```python
from build123d import *

# Parameters (mm, degrees)
SKETCH1_W                        = 12.7
SKETCH1_H                        = 6.0198
BOSS_EXTRUDE1_DEPTH              = 5.7658
SKETCH13_R                       = 0.635
CUT_EXTRUDE2_DEPTH               = 5.7658
CHAMFER1_SIZE                    = 50.8
F_4_CLEARANCE_HOLE1_D            = 2.9464
F_4_CLEARANCE_HOLE1_DEPTH        = 6.35
F_4_CLEARANCE_HOLE1_TIP          = 0.885187864
F_3_8_0_375_DIAMETER_HOLE1_D     = 9.525
F_3_8_0_375_DIAMETER_HOLE1_DEPTH = 6.35
F_3_8_0_375_DIAMETER_HOLE1_TIP   = 2.861598698
CUT_EXTRUDE3_REACH               = 234.708
FILLET3_R                        = 6.35
CUT_EXTRUDE4_REACH               = 234.708
CUT_EXTRUDE5_REACH               = 234.708
SKETCH26_W                       = 2.9591
SKETCH26_H                       = 9.525
CUT_EXTRUDE6_REACH               = 234.708
SKETCH29_W                       = 65.024
SKETCH29_H                       = 36.83
FILLET5_R                        = 6.35
CUT_EXTRUDE9_REACH               = 234.708
SKETCH32_W                       = 9.525
SKETCH32_H                       = 2.9591
CUT_EXTRUDE10_REACH              = 234.708
CHAMFER2_SIZE                    = 19.05
CUT_EXTRUDE11_START              = -5.7658
CUT_EXTRUDE11_DEPTH              = 5.7658
CUT_EXTRUDE12_REACH              = 234.708
SKETCH36_W                       = 57.277
SKETCH36_H                       = 36.83
FILLET7_R                        = 2.54
FILLET8_R                        = 6.35
CUT_EXTRUDE13_REACH              = 234.708
SKETCH37_W                       = 9.525
SKETCH37_H                       = 2.9591
F_4_CLEARANCE_HOLE2_D            = 2.9464
F_4_CLEARANCE_HOLE2_DEPTH        = 5.7658
SKETCH38_W                       = 50.8
SKETCH38_H                       = 19.05
CUT_EXTRUDE14_DEPTH              = 233.70795425
FILLET9_R                        = 6.35
TAP_DRILL_FOR_4_HELICOIL1_D      = 3.9878


with BuildPart() as part:
    # Sketch1 → Boss-Extrude1 (new body)
    with BuildSketch(Plane.XY):
        Polygon((-25.4, 0), (25.4, 0), (25.4, -6.35), (38.1, -6.35), (38.1, 0), (44.45, 0), (44.45, 205.2008), (-109.601, 205.2008), (-109.601, 135.3508), (-44.45, 135.3508), (-44.45, 0), (-38.1, 0), (-38.1, -6.35), (-25.4, -6.35), align=None)
        with Locations((12.7, 9.3599)):
            Rectangle(SKETCH1_W, SKETCH1_H, mode=Mode.SUBTRACT)
        with Locations((-12.7, 9.3599)):
            Rectangle(SKETCH1_W, SKETCH1_H, mode=Mode.SUBTRACT)
    extrude(amount=BOSS_EXTRUDE1_DEPTH)

    # Sketch13 → Cut-Extrude2 (cut)
    with BuildSketch(Plane.XY):
        with Locations((-19.05, 12.3698)):
            Circle(SKETCH13_R)
    cut_extrude2 = extrude(amount=CUT_EXTRUDE2_DEPTH, mode=Mode.SUBTRACT)

    # Sketch-Pattern1: Cut-Extrude2 at 11 more places
    with Locations((12.7, 0, 0), (12.7, -6.0198, 0), (0, -6.0198, 0), (25.4, 0, 0), (38.1, 0, 0), (38.1, -6.0198, 0), (25.4, -6.0198, 0), (57.15, -12.3698, 0), (44.45, -12.3698, 0), (-6.35, -12.3698, 0), (-19.05, -12.3698, 0)):
        add(cut_extrude2, mode=Mode.SUBTRACT)

    # Chamfer1
    chamfer1_edges = [part.edges().sort_by_distance(p)[0] for p in [
        (44.45, 205.2008, 2.8829),
    ]]
    chamfer(chamfer1_edges, length=CHAMFER1_SIZE)

    # 4 Clearance Hole1
    with Locations(Plane.XY.offset(5.7658)):
        with Locations((-31.75, 3.175), (31.75, 3.175), (0, 3.175)):
            Hole(F_4_CLEARANCE_HOLE1_D / 2, depth=F_4_CLEARANCE_HOLE1_DEPTH)
            with Locations((0, 0, -(F_4_CLEARANCE_HOLE1_DEPTH + F_4_CLEARANCE_HOLE1_TIP / 2))):  # 118° drill point
                Cone(0, F_4_CLEARANCE_HOLE1_D / 2, F_4_CLEARANCE_HOLE1_TIP, mode=Mode.SUBTRACT)

    # 3_8 _0.375_ Diameter Hole1
    with Locations(Plane.XY.offset(5.7658)):
        with Locations((-100.076, 144.8758), (-100.076, 195.6758)):
            Hole(F_3_8_0_375_DIAMETER_HOLE1_D / 2, depth=F_3_8_0_375_DIAMETER_HOLE1_DEPTH)
            with Locations((0, 0, -(F_3_8_0_375_DIAMETER_HOLE1_DEPTH + F_3_8_0_375_DIAMETER_HOLE1_TIP / 2))):  # 118° drill point
                Cone(0, F_3_8_0_375_DIAMETER_HOLE1_D / 2, F_3_8_0_375_DIAMETER_HOLE1_TIP, mode=Mode.SUBTRACT)

    # Sketch24 → Cut-Extrude3 (cut, up to next)
    with BuildSketch(Plane.XY.offset(5.7658), mode=Mode.PRIVATE) as cut_extrude3_sk1:
        Polygon((31.75, 167.1008), (31.75, 16.002), (44.45, 16.002), (44.45, 154.4008), align=None)
    cut_extrude3_tool1 = extrude(cut_extrude3_sk1.sketch, amount=-CUT_EXTRUDE3_REACH, mode=Mode.PRIVATE) & part.part
    add(cut_extrude3_tool1.solids().sort_by_distance((38.007144, 88.422828, 5.7658))[0], mode=Mode.SUBTRACT)

    # Fillet3
    fillet3_edges = [part.edges().sort_by_distance(p)[0] for p in [
        (31.75, 16.002, 2.8829),
    ]]
    fillet(fillet3_edges, radius=FILLET3_R)

    # Sketch25 → Cut-Extrude4 (cut, up to next)
    with BuildSketch(Plane.XY.offset(5.7658), mode=Mode.PRIVATE) as cut_extrude4_sk1:
        with BuildLine():
            ThreePointArc((-20.441531288, 134.8428), (-19.812, 144.8758), (-20.441531288, 154.9088))
            ThreePointArc((-20.441531288, 154.9088), (-24.981656286, 158.432924998), (-28.505781284, 153.8928))
            ThreePointArc((-28.505781284, 153.8928), (-27.94, 144.8758), (-28.505781284, 135.8588))
            ThreePointArc((-28.505781284, 135.8588), (-24.981656286, 131.318675002), (-20.441531288, 134.8428))
        make_face()
    cut_extrude4_tool1 = extrude(cut_extrude4_sk1.sketch, amount=-CUT_EXTRUDE4_REACH, mode=Mode.PRIVATE) & part.part
    # Sketch25 → Cut-Extrude4 (cut, up to next)
    with BuildSketch(Plane.XY.offset(5.7658), mode=Mode.PRIVATE) as cut_extrude4_sk2:
        with BuildLine():
            ThreePointArc((17.359640569, 130.0803), (18.288, 144.8758), (17.359640569, 159.6713))
            ThreePointArc((17.359640569, 159.6713), (12.819515571, 163.195424998), (9.295390572, 158.6553))
            ThreePointArc((9.295390572, 158.6553), (10.16, 144.8758), (9.295390572, 131.0963))
            ThreePointArc((9.295390572, 131.0963), (12.819515571, 126.556175002), (17.359640569, 130.0803))
        make_face()
    cut_extrude4_tool2 = extrude(cut_extrude4_sk2.sketch, amount=-CUT_EXTRUDE4_REACH, mode=Mode.PRIVATE) & part.part
    add(cut_extrude4_tool1.solids().sort_by_distance((-24.175106, 144.8758, 5.7658))[0], mode=Mode.SUBTRACT)
    add(cut_extrude4_tool2.solids().sort_by_distance((13.816141, 144.8758, 5.7658))[0], mode=Mode.SUBTRACT)

    # Sketch26 → Cut-Extrude5 (cut, up to next)
    with BuildSketch(Plane.XY.offset(5.7658), mode=Mode.PRIVATE) as cut_extrude5_sk1:
        with Locations((9.35355, 61.214)):
            Rectangle(SKETCH26_W, SKETCH26_H)
    cut_extrude5_tool1 = extrude(cut_extrude5_sk1.sketch, amount=-CUT_EXTRUDE5_REACH, mode=Mode.PRIVATE) & part.part
    # Sketch26 → Cut-Extrude5 (cut, up to next)
    with BuildSketch(Plane.XY.offset(5.7658), mode=Mode.PRIVATE) as cut_extrude5_sk2:
        with Locations((-19.00555, 61.214)):
            Rectangle(SKETCH26_W, SKETCH26_H)
    cut_extrude5_tool2 = extrude(cut_extrude5_sk2.sketch, amount=-CUT_EXTRUDE5_REACH, mode=Mode.PRIVATE) & part.part
    add(cut_extrude5_tool1.solids().sort_by_distance((9.35355, 61.214, 5.7658))[0], mode=Mode.SUBTRACT)
    add(cut_extrude5_tool2.solids().sort_by_distance((-19.00555, 61.214, 5.7658))[0], mode=Mode.SUBTRACT)

    # Sketch29 → Cut-Extrude6 (cut, up to next)
    with BuildSketch(Plane.XY.offset(5.7658), mode=Mode.PRIVATE) as cut_extrude6_sk1:
        with Locations((-0.762, 186.7858)):
            Rectangle(SKETCH29_W, SKETCH29_H)
    cut_extrude6_tool1 = extrude(cut_extrude6_sk1.sketch, amount=-CUT_EXTRUDE6_REACH, mode=Mode.PRIVATE) & part.part
    add(cut_extrude6_tool1.solids().sort_by_distance((-0.762, 186.7858, 5.7658))[0], mode=Mode.SUBTRACT)

    # Fillet5
    fillet5_edges = [part.edges().sort_by_distance(p)[0] for p in [
        (-33.274, 168.3708, 2.8829),
    ]]
    fillet(fillet5_edges, radius=FILLET5_R)

    # Sketch32 → Cut-Extrude9 (cut, up to next)
    with BuildSketch(Plane.XY.offset(5.7658), mode=Mode.PRIVATE) as cut_extrude9_sk1:
        with Locations((20.6375, 166.0975)):
            Rectangle(SKETCH32_W, SKETCH32_H)
    cut_extrude9_tool1 = extrude(cut_extrude9_sk1.sketch, amount=-CUT_EXTRUDE9_REACH, mode=Mode.PRIVATE) & part.part
    add(cut_extrude9_tool1.solids().sort_by_distance((20.6375, 166.0975, 5.7658))[0], mode=Mode.SUBTRACT)

    # Sketch31 → Cut-Extrude10 (cut, up to next)
    with BuildSketch(Plane.XY.offset(5.7658), mode=Mode.PRIVATE) as cut_extrude10_sk1:
        with BuildLine():
            Line((-12.446, 77.0763), (-12.446, 115.1763))
            ThreePointArc((-12.446, 115.1763), (-4.826, 122.7963), (2.794, 115.1763))
            Line((2.794, 115.1763), (2.794, 77.0763))
            ThreePointArc((2.794, 77.0763), (-4.826, 69.4563), (-12.446, 77.0763))
        make_face()
    cut_extrude10_tool1 = extrude(cut_extrude10_sk1.sketch, amount=-CUT_EXTRUDE10_REACH, mode=Mode.PRIVATE) & part.part
    add(cut_extrude10_tool1.solids().sort_by_distance((-4.826, 96.1263, 5.7658))[0], mode=Mode.SUBTRACT)

    # Chamfer2
    chamfer2_edges = [part.edges().sort_by_distance(p)[0] for p in [
        (-44.45, 135.3508, 2.8829),
    ]]
    chamfer(chamfer2_edges, length=CHAMFER2_SIZE)

    # Sketch35 → Cut-Extrude11 (cut)
    with BuildSketch(Plane.XY.offset(5.7658).offset(CUT_EXTRUDE11_START)):
        Polygon((31.75, 63.5), (15.875, 63.5), (15.875, 126.5243), (9.263515571, 126.5243), (9.263515571, 168.3708), (31.75, 168.3708), align=None)
    extrude(amount=CUT_EXTRUDE11_DEPTH, mode=Mode.SUBTRACT)

    # Sketch36 → Cut-Extrude12 (cut, up to next)
    with BuildSketch(Plane.XY.offset(5.7658), mode=Mode.PRIVATE) as cut_extrude12_sk1:
        with Locations((-55.5625, 186.7858)):
            Rectangle(SKETCH36_W, SKETCH36_H)
    cut_extrude12_tool1 = extrude(cut_extrude12_sk1.sketch, amount=-CUT_EXTRUDE12_REACH, mode=Mode.PRIVATE) & part.part
    add(cut_extrude12_tool1.solids().sort_by_distance((-55.5625, 186.7858, 5.7658))[0], mode=Mode.SUBTRACT)

    # Fillet7
    fillet7_edges = [part.edges().sort_by_distance(p)[0] for p in [
        (15.875, 63.5, 2.8829),
        (9.263515571, 126.5243, 2.8829),
    ]]
    fillet(fillet7_edges, radius=FILLET7_R)

    # Fillet8
    fillet8_edges = [part.edges().sort_by_distance(p)[0] for p in [
        (-84.201, 168.3708, 2.8829),
    ]]
    fillet(fillet8_edges, radius=FILLET8_R)

    # Sketch37 → Cut-Extrude13 (cut, up to next)
    with BuildSketch(Plane.XY.offset(5.7658), mode=Mode.PRIVATE) as cut_extrude13_sk1:
        with Locations((-46.298984429, 165.30375)):
            Rectangle(SKETCH37_W, SKETCH37_H)
    cut_extrude13_tool1 = extrude(cut_extrude13_sk1.sketch, amount=-CUT_EXTRUDE13_REACH, mode=Mode.PRIVATE) & part.part
    add(cut_extrude13_tool1.solids().sort_by_distance((-46.298984, 165.30375, 5.7658))[0], mode=Mode.SUBTRACT)

    # 4 Clearance Hole2
    with Locations(Plane.XY.offset(5.7658)):
        with Locations((-24.1681, 61.214), (14.5161, 61.214), (20.6375, 117.5708), (-100.076, 182.9758), (-100.076, 157.5758), (-62.173984429, 165.30375), (-30.423984429, 165.30375)):
            Hole(F_4_CLEARANCE_HOLE2_D / 2, depth=F_4_CLEARANCE_HOLE2_DEPTH)

    # Sketch38 → Cut-Extrude14 (cut, through all)
    with BuildSketch(Plane.XY.offset(5.7658)):
        with Locations((-6.35, 34.5948)):
            Rectangle(SKETCH38_W, SKETCH38_H)
    extrude(amount=-CUT_EXTRUDE14_DEPTH, mode=Mode.SUBTRACT)

    # Fillet9
    fillet9_edges = [part.edges().sort_by_distance(p)[0] for p in [
        (19.05, 44.1198, 2.8829),
        (19.05, 25.0698, 2.8829),
        (-31.75, 25.0698, 2.8829),
        (-31.75, 44.1198, 2.8829),
    ]]
    fillet(fillet9_edges, radius=FILLET9_R)

    # Tap Drill for _4 Helicoil1 (through all)
    with Locations(Plane.XY.offset(5.7658)):
        with Locations((-92.456, 165.7038), (-83.031, 165.7038)):
            Hole(TAP_DRILL_FOR_4_HELICOIL1_D / 2)


solid = part.part
```
Verification items for the finished model (mm, model axes). A direction names the side the tool comes from. Coordinates: 2 decimals unless noted, no trailing zeros. Loops run counter-clockwise (first coordinate to the right, second up) from the corner with the lowest first, then second, coordinate; pieces in that order, holes last. Notation, with made-up numbers: (52, -34) -> (97, -34) arc R11 cw to (97, -23) -> close; hole circle Ø9 at (-14, 73.5). An arc over 180 degrees is marked (long way). Answer in a Markdown table with one row per item.
1) Section check B-B (x = -73). Record the cut outline in (y, z), and give its area (3 significant figures).
The answers:
| item | result |
|---|---|
| outline | (135.35, 0) -> (168.37, 0) -> (168.37, 5.77) -> (135.35, 5.77) -> close |
| area | 190 mm2 |
2) Section check C-C (z = 2.35). Give the number of separate pieces and of enclosed holes in the cut face, and give its area (3 significant figures).
The answers:
| item | result |
|---|---|
| separate pieces | 1 |
| enclosed holes | 21 |
| area | 12,200 mm2 |
3) Section check A-A (y = 110.5). Record the cut outline in (x, z) (3 decimals), and give its area (3 significant figures).
The answers:
| item | result |
|---|---|
| outline | (-44.45, 0) -> (-12.446, 0) -> (-12.446, 5.766) -> (-44.45, 5.766) -> close; (2.794, 0) -> (15.875, 0) -> (15.875, 5.766) -> (2.794, 5.766) -> close |
| area | 260 mm2 |
4) Scan lines: line 1 along Y through (x, z) = (-16.5, 4.1); line 2 along X through (y, z) = (110, 0.9) (3 decimals); line 3 along Y through (x, z) = (-21, 3.4). Record each from-to range of solid material in increasing order. Write a range as from..to.
The answers:
| item | result |
|---|---|
| line 1 | y = 0..6.35, 12.37..25.07, 44.12..168.37 |
| line 2 | x = -44.45..-12.446, 2.794..15.875 |
| line 3 | y = 0..25.07, 44.12..133.24, 156.51..168.37 |
5) Draft check along X on faces 1 (the face through (32, -6.35, 3)), 2 (the face through (-93.376, 163.935, 2.843)), 3 (the face through (-53.84, 125.69, 2.84)). Enter one of: released by +X, released by -X, zero draft, split by the parting line, or undercut.
The answers:
| item | result |
|---|---|
| face 1 | zero draft |
| face 2 | undercut |
| face 3 | released by -X |
6) Depth check by flat-ended pin: P1, Ø1.7, axis at y = 94, z = 3.5, coming from the +X side (3 decimals); P2, Ø4, axis at x = 14.52, y = 61.21, coming from the -Z side; P3, Ø1.7, axis at x = -14, z = 3.5, coming from the -Y side; P4, Ø3, axis at y = 29.5, z = 5, coming from the -X side. Enter the tip coordinate at first touch or a pass-through.
The answers:
| item | result |
|---|---|
| P1 | stops at x = 15.875 |
| P2 | stops at z = 0 |
| P3 | stops at y = 0 |
| P4 | stops at x = -44.45 |
7) Access from +Z, -Z, +X, -X, +Y, -Y to the whole of each face (thin tool, end or side, straight path). Record for faces 4 (the face through (-87, 135.351, 3)), 5 (the face through (-20.485, 61, 3)), 6 (the face through (44.45, 8, 3)), 7 (the face through (31.75, 43, 3)).
The answers:
| item | result |
|---|---|
| face 4 | +Z, -Z, -X, -Y |
| face 5 | +Z, -Z |
| face 6 | +Z, -Z, +X, +Y, -Y |
| face 7 | +Z, -Z, +X, +Y |
